CAD build for the part. Positions are in the model's coordinates, mm. Face numbers are marked on the shaded views. A direction names the side the tool comes from. Give positions to 0.01 mm unless a question says otherwise; leave off trailing zeros. Write each loop counter-clockwise with the first axis right and the second up, starting at its lowest first coordinate (ties: lowest second). Pieces come first, ordered by that corner, then holes. Notation, with made-up numbers: (43, 80) - (48, 80) arc R22 cw to (48, 108) - close; hole circle Ø11 at (47, 59). An arc over 180 degrees is marked (long way). Answer as a JSON object with one key per item and string values.
from build123d import *

# Parameters (mm, degrees)
BOSS_EXTRUDE1_DEPTH = 5.334
SKETCH4_W           = 21.336
SKETCH4_H           = 1.651


with BuildPart() as part:
    # Sketch2 → Revolve1 (revolve)
    with BuildSketch(Plane(origin=(0, 0, 0), x_dir=(0, 0, -1), z_dir=(1, 0, 0))):
        Polygon((5.1308, 3.175), (5.1308, 3.048), (6.582416642, 3.175), (16.002, 3.175), (16.002, 0), (0, 0), (0, 3.175), align=None)
    revolve(axis=Axis((0, 0, -16.002), (0, 0, 1)))

    # Sketch3 → Boss-Extrude1 (add)
    with BuildSketch(Plane(origin=(0, 0, -16.002), x_dir=(-1, 0, 0), z_dir=(0, 0, -1))):
        Polygon((0, 8.248891971), (-7.14375, 4.124445986), (-7.14375, -4.124445986), (0, -8.248891971), (7.14375, -4.124445986), (7.14375, 4.124445986), align=None)
    extrude(amount=BOSS_EXTRUDE1_DEPTH)

    # Sketch4 → Cut-Revolve1 (revolve, cut)
    with BuildSketch(Plane(origin=(0, 0, 0), x_dir=(0, 0, -1), z_dir=(1, 0, 0))):
        Polygon((16.002, 8.248891971), (16.002, 7.14375), (16.640054014, 8.248891971), (20.697945986, 8.248891971), (21.336, 7.14375), (21.336, 8.248891971), (21.336, 9.354033942), (16.002, 9.354033942), align=None)
        with Locations((10.668, 0.8255)):
            Rectangle(SKETCH4_W, SKETCH4_H)
    revolve(axis=Axis((0, 0, 0), (0, 0, -1)), mode=Mode.SUBTRACT)


with BuildPart() as body_2:
    # Sketch5 → Revolve2 (revolve)
    with BuildSketch(Plane(origin=(0, 0, 0), x_dir=(0, 0, -1), z_dir=(1, 0, 0))):
        Polygon((20.45716, 0), (35.56, 0), (35.56, 6.38777167), (20.45716, 6.858), align=None)
    revolve(axis=Axis((0, 0, -20.45716), (0, 0, -1)))


with BuildPart() as part_1:
    add(part.part)

    # Combine1: union body 2
    add(body_2.part)

    # Sketch8 → Cut-Revolve2 (revolve, cut)
    with BuildSketch(Plane(origin=(0, 0, 0), x_dir=(0, 0, -1), z_dir=(1, 0, 0))):
        Polygon((35.56, 5.318470859), (34.33794193, 6.540528929), (35.56, 6.540528929), align=None)
        Polygon((35.56, 4.6228), (20.45716, 4.6228), (17.67950153, 0), (35.56, 0), align=None)
    revolve(axis=Axis((0, 0, 0), (0, 0, -1)), mode=Mode.SUBTRACT)


solid = part_1.part
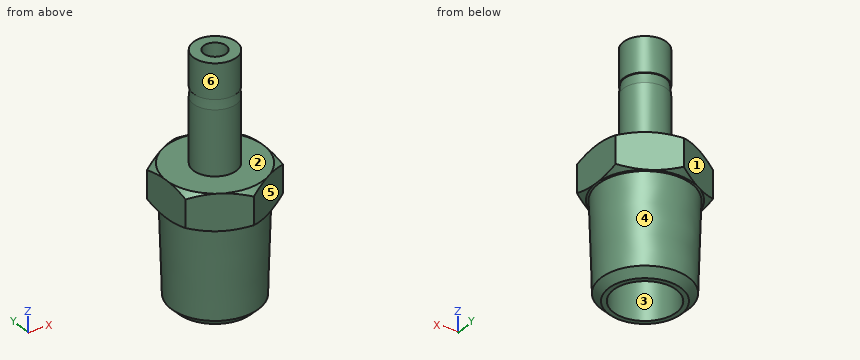
Item 1: Which spindle directions (+Z, -Z, +X, -X, +Y, -Y) get a long thin tool onto all of the face, cutting with end or side? Do the marked faces 4, 5 and 6. Say none if no direction does.
Entries:
{"face 4": "-Z", "face 5": "+Z, -Z, +X, -Y", "face 6": "+Z"}
Item 2: Cut at B-B (z = -33). Give the cut face in (x, y), and give its area (3 significant figures).
Entries:
{"outline": "circle Ø12.93 at (0, 0); hole circle Ø9.25 at (0, 0)", "area": "64.3 mm2"}
Item 3: Probe line 1 (X direction, y = 0, z = -10.5) (3 decimals); line 2 (X direction, y = 0, z = -25.75); line 3 (Y direction, x = 0.25, z = -9). List the from-to ranges inside material, lowest first. Write a range as from..to.
Entries:
{"line 1": "-3.175..-1.651, 1.651..3.175", "line 2": "-6.69..-4.62, 4.62..6.69", "line 3": "-3.17..-1.63, 1.63..3.17"}
Item 4: Cut at A-A (z = -7). Give the cut face in (x, y) (3 decimals).
Entries:
{"outline": "circle Ø6.35 at (0, 0); hole circle Ø3.302 at (0, 0)"}
Item 5: Flat gauge pins, fed straight in: P1, Ø4, axis at x = -2, z = -4, coming from the +Y side (3 decimals); P2, Ø2, axis at x = 1, z = -11, coming from the -Y side (3 decimals); P3, Ø3, axis at y = 4, z = -13.5, coming from the +X side. Where does each tip first touch, or does it go through?
Entries:
{"P1": "y = 3.175", "P2": "y = -3.175", "P3": "x = 1.96"}
Item 6: Mould opens along X. For the marked faces 1, 2 and 3 say: +X half, -X half, draft (parallel to the pull), parting line (faces both ways), or undercut.
Entries:
{"face 1": "-X half", "face 2": "draft", "face 3": "undercut"}
